Job drawing, mm, ordinate dimensions from the low corner. One solid piece. Coordinates: 2 decimals unless noted, no trailing zeros. Write each loop counter-clockwise with the first axis right and the second up, starting at its lowest first coordinate (ties: lowest second). Pieces come first, ordered by that corner, then holes. Notation, with made-up numbers: (86.25, -32.75) - (93.25, -32.75) arc R16 ccw to (93.25, -12.75) - close; hole circle Ø6 at (-9.5, 31). An arc over 180 degrees is marked (long way). Use a Markdown table: item, result.
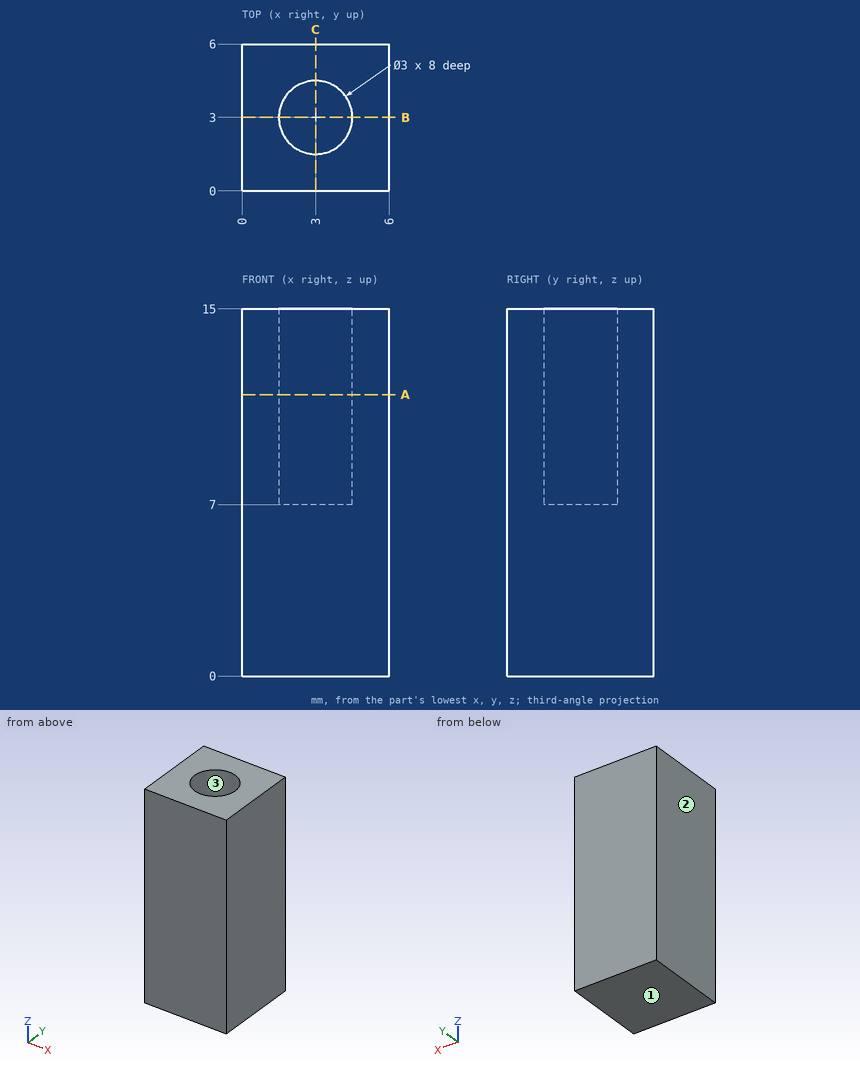
Item 1: Band-saw the part on B-B, the plane y = 3. Give the cut face in (x, z).
From the geometry:
| item | result |
|---|---|
| outline | (0, 0) - (6, 0) - (6, 15) - (4.5, 15) - (4.5, 7) - (1.5, 7) - (1.5, 15) - (0, 15) - close |
Item 2: Band-saw the part on A-A, the plane z = 11.5. Give the cut face in (x, y).
From the geometry:
| item | result |
|---|---|
| outline | (0, 0) - (6, 0) - (6, 6) - (0, 6) - close; hole circle Ø3 at (3, 3) |
Item 3: Two-plate mould, pull along X, no slides. Class the marked faces 1, 2 and 3: pulls with the +X half, pulls with the -X half, needs draft (parallel to the pull), parting line crosses it, or undercut.
From the geometry:
| item | result |
|---|---|
| face 1 | needs draft |
| face 2 | pulls with the -X half |
| face 3 | undercut |
Item 4: Drill centre lines: probe 1 along Y at (x, z) = (3, 11); probe 2 along Z at (x, y) = (3.2, 2.85); probe 3 along X at (y, z) = (1.9, 13.25). Where is each one in solid material? Low to high.
From the geometry:
| item | result |
|---|---|
| probe 1 | 0 to 1.5, 4.5 to 6 |
| probe 2 | 0 to 7 |
| probe 3 | 0 to 1.98, 4.02 to 6 |
Item 5: Drop a flat-ended pin along its axis: P1, Ø0.9, axis at x = 3, y = 3.5, coming from the +Z side. Give the stop position or say it passes through.
From the geometry:
| item | result |
|---|---|
| P1 | z = 7 |
